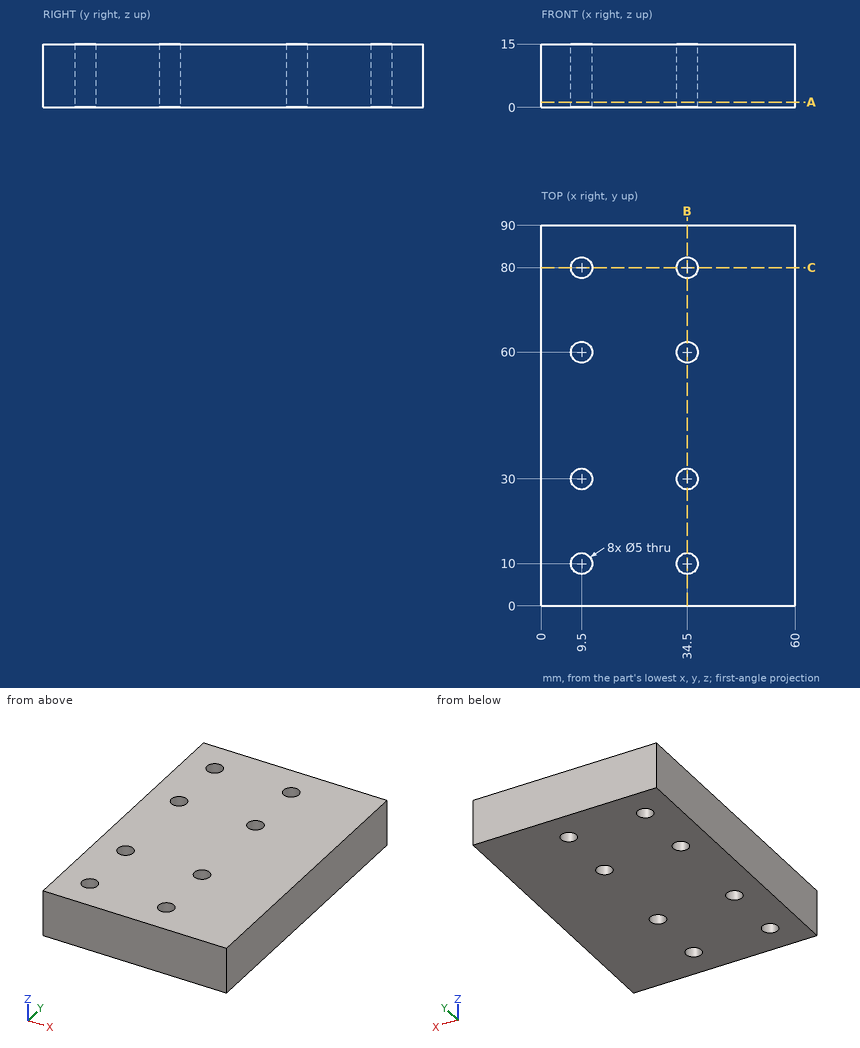
Here's the drawing with two shaded views (mm, measured from the low corner). I have some questions. Round coordinates to 2 decimals unless told otherwise and drop trailing zeros. Write each loop counter-clockwise with the first axis right and the second up, starting at its lowest first coordinate (ties: lowest second). Pieces come first, ordered by that corner, then holes. Notation, with made-up numbers: M -2,-27 L 55,-27 A6 ccw 55,-20 Z; hole C 36.25,-20 d11. An arc over 180 degrees is marked long. Answer in a Markdown table with one row per item. Add a question column.
Q1. Imagine slicing it at C-C (y = 80). Please give me the cut outline in (x, z), then the cut area to 3 significant figures.
Q2. Imagine slicing it at B-B (x = 34.5). Please give me the cut outline in (y, z), then the cut area to 3 significant figures.
Q3. Imagine slicing it at A-A (z = 1.25). Give the number of separate pieces and of enclosed holes in the cut face, then the cut area to 3 significant figures.
Q4. Will this pin go through, and if not, where does the flat tip stop? pin 1 Ø3 at (x, y) = (34.5, 80) entering from -Z.
Q5. If I drill on line 1 (Y direction, x = 9.5, z = 7.5); line 2 (X direction, y = 11, z = 9); line 3 (Y direction, x = 11.5, z = 1), over which ranges is the centre line in solid material (lowest first)? Write a range as from..to.
Values:
| question | item | result |
|---|---|---|
| 1 | outline | M 0,0 L 7,0 L 7,15 L 0,15 Z; M 12,0 L 32,0 L 32,15 L 12,15 Z; M 37,0 L 60,0 L 60,15 L 37,15 Z |
| 1 | area | 750 mm^2 |
| 2 | outline | M 0,0 L 7.5,0 L 7.5,15 L 0,15 Z; M 12.5,0 L 27.5,0 L 27.5,15 L 12.5,15 Z; M 32.5,0 L 57.5,0 L 57.5,15 L 32.5,15 Z; M 62.5,0 L 77.5,0 L 77.5,15 L 62.5,15 Z; M 82.5,0 L 90,0 L 90,15 L 82.5,15 Z |
| 2 | area | 1,050 mm^2 |
| 3 | separate pieces | 1 |
| 3 | enclosed holes | 8 |
| 3 | area | 5,240 mm^2 |
| 4 | pin 1 | through |
| 5 | line 1 | 0..7.5, 12.5..27.5, 32.5..57.5, 62.5..77.5, 82.5..90 |
| 5 | line 2 | 0..7.21, 11.79..32.21, 36.79..60 |
| 5 | line 3 | 0..8.5, 11.5..28.5, 31.5..58.5, 61.5..78.5, 81.5..90 |
